from build123d import *

# Parameters (mm, degrees)
SKETCH_1_R               = 6.65
EXTRUDE_1_DEPTH          = 20
SKETCH_2_R               = 1.5
CUT_EXTRUDE_1_DEPTH      = 35.073450075
SKETCH_3_R               = 1.45
CUT_EXTRUDE_2_DEPTH      = 10
PATTERN_CIRCULAR_1_COUNT = 2
PATTERN_CIRCULAR_1_ANGLE = 90
F_1_THE_OTHER_WAY_COUNT  = 2
F_1_THE_OTHER_WAY_ANGLE  = 90
SKETCH_4_R               = 4.65
EXTRUDE_2_DEPTH          = 2
FILLET_1_R               = 2


with BuildPart() as part:
    # 草图1 → 凸台-拉伸1 (new body)
    with BuildSketch(Plane(origin=(0, 0, 0), x_dir=(1, 0, 0), z_dir=(0, 1, 0))):
        with BuildLine():
            Line((-11, 0), (-11, -8))
            Line((-11, -8), (-20, -8))
            Line((-20, -8), (-20, -13))
            Line((-20, -13), (20, -13))
            Line((20, -13), (20, -8))
            Line((20, -8), (11, -8))
            Line((11, -8), (11, 0))
            ThreePointArc((11, 0), (0, 11), (-11, 0))
        make_face()
        with Locations(Location((0, 0, 0), (0, 0, 270))):
            Circle(SKETCH_1_R, mode=Mode.SUBTRACT)
    extrude(amount=EXTRUDE_1_DEPTH)

    # 草图2 → 切除-拉伸1 (cut, through all)
    with BuildSketch(Plane(origin=(0, 0, 8), x_dir=(-1, 0, 0), z_dir=(0, 0, -1))):
        with Locations((15.5, 5)):
            Circle(SKETCH_2_R)
        with Locations(Location((15.5, 15, 0), (0, 0, 180))):
            Circle(SKETCH_2_R)
        with Locations((-15.5, 15)):
            Circle(SKETCH_2_R)
        with Locations(Location((-15.5, 5, 0), (0, 0, 180))):
            Circle(SKETCH_2_R)
    extrude(amount=-CUT_EXTRUDE_1_DEPTH, mode=Mode.SUBTRACT)

    # 草图3 → 切除-拉伸2 (cut)
    with BuildSketch(Plane(origin=(0, 0, -11), x_dir=(-1, 0, 0), z_dir=(0, 0, -1))):
        with Locations((0, 6)):
            Circle(SKETCH_3_R)
        with Locations((0, 14)):
            Circle(SKETCH_3_R)
    cut_extrude_2 = extrude(amount=-CUT_EXTRUDE_2_DEPTH, mode=Mode.SUBTRACT)

    # 阵列(圆周)1: 切除-拉伸2 ×2 about axis
    pattern_circular_1_axis = Axis((0, 20, 0), (0, -1, 0))
    for i in range(1, PATTERN_CIRCULAR_1_COUNT):
        add(cut_extrude_2.rotate(pattern_circular_1_axis, i * PATTERN_CIRCULAR_1_ANGLE / (PATTERN_CIRCULAR_1_COUNT - 1)), mode=Mode.SUBTRACT)

    # 1 the other way: 切除-拉伸2 ×2 about axis
    f_1_the_other_way_axis = Axis((0, 20, 0), (0, 1, 0))
    for i in range(1, F_1_THE_OTHER_WAY_COUNT):
        add(cut_extrude_2.rotate(f_1_the_other_way_axis, i * F_1_THE_OTHER_WAY_ANGLE / (F_1_THE_OTHER_WAY_COUNT - 1)), mode=Mode.SUBTRACT)

    # 草图4 → 凸台-拉伸2 (add)
    with BuildSketch(Plane(origin=(0, 20, 0), x_dir=(1, 0, 0), z_dir=(0, 1, 0))):
        with BuildLine():
            Line((20, -8), (11, -8))
            Line((11, -8), (11, 0))
            ThreePointArc((11, 0), (0, 11), (-11, 0))
            Line((-11, 0), (-11, -8))
            Line((-11, -8), (-20, -8))
            Line((-20, -8), (-20, -13))
            Line((-20, -13), (20, -13))
            Line((20, -13), (20, -8))
        make_face()
        with Locations(Location((0, 0, 0), (0, 0, 270))):
            Circle(SKETCH_4_R, mode=Mode.SUBTRACT)
    extrude(amount=EXTRUDE_2_DEPTH)

    # 圆角1
    fillet_1_edges = [part.edges().sort_by_distance(p)[0] for p in [
        (20, 0, 10.5),
        (-20, 0, 10.5),
        (20, 22, 10.5),
        (-20, 22, 10.5),
    ]]
    fillet(fillet_1_edges, radius=FILLET_1_R)


solid = part.part
The model under review builds one solid part; all positions refer to its coordinate system, in mm. A direction names the side the tool comes from. Give positions to 0.01 mm unless a question says otherwise; leave off trailing zeros. Order: outer loops, then holes, each group sorted by start corner. A loop starts at its lowest first (then second) coordinate and runs counter-clockwise, first axis right, second up. Notation, with made-up numbers: M 45,41.5 L 88,41.5 A16 ccw 88,68.5 Z; hole C 19.5,-29 d3. An arc over 180 degrees is marked long. One line per question, with ' | ' between items. Start each with the question number.
1) For faces 5 (the face through (-15, 11, 8)), 6 (the face through (11, 11, 4)), 7 (the face through (1.397, 20.986, 4.435)), 8 (the face through (0.189, 15.438, -8.777)), 9 (the face through (-5, 20, 1)), list the 3-axis set-ups (+Z, -Z, +X, -X, +Y, -Y) from which the entire face can be reached by the end or side of a thin tool; tool diameter is ignored.
2) Consider section D-D, the plane x = 15.5. Give the boundary of the cut face in (y, z), then the cut area to 3 significant figures.
3) Consider section A-A, the plane x = 0. Give the boundary of the cut face in (y, z), then the cut area to 3 significant figures.
4) Consider section C-C, the plane y = 12. Give the boundary of the cut face in (x, z).
5) Consider section B-B, the plane z = 9. Give the boundary of the cut face in (x, y).
6) Clearance check with flat-ended pins moving along their axes: P1, Ø4, axis at x = -1.5, z = -1, coming from the -Y side; P2, Ø3.5, axis at x = -15.5, y = 5, coming from the -Z side; P3, Ø4, axis at x = 10.5, y = 18, coming from the -Z side; P4, Ø2, axis at y = 8, z = 1.5, coming from the +X side. State where each tip first meets the part, or that it passes through.
7) Mouldability with a two-part tool opening along X and no side actions: class faces 1 (the face through (-8.774, 7.438, -0.189)), 2 (the face through (-14, 5, 10)), 3 (the face through (19.4, 0.57, 10.46)), 4 (the face through (-5.9, 9.86, 3.07)) as pulls with the +X half, pulls with the -X half, needs draft (parallel to the pull), parting line crosses it, or undercut.
8) Wall thickness on L1, parallel to Y at x = -15.5, z = 9.4; L2, parallel to Y at x = 0, z = -8.25; L3, parallel to X at y = 3.75, z = 0.25: over which ranges is each line inside the solid? List them lowest first. Write a range as from..to.
Found:
1) face 5: -Z, -X, +Y, -Y | face 6: -Z, +X, +Y, -Y | face 7: +Y, -Y | face 8: -Z | face 9: -Y
2) outline: M 0,8 L 3.5,8 L 3.5,13 L 0,13 Z; M 6.5,8 L 13.5,8 L 13.5,13 L 6.5,13 Z; M 16.5,8 L 22,8 L 22,13 L 16.5,13 Z | area: 80.0 mm²
3) outline: M 0,-11 L 4.55,-11 L 4.55,-6.65 L 0,-6.65 Z; M 0,6.65 L 20,6.65 L 20,4.65 L 22,4.65 L 22,13 L 0,13 Z; M 7.45,-11 L 12.55,-11 L 12.55,-6.65 L 7.45,-6.65 Z; M 15.45,-11 L 22,-11 L 22,-4.65 L 20,-4.65 L 20,-6.65 L 15.45,-6.65 Z | area: 218 mm²
4) outline: M -20,8 L -11,8 L -11,0 A11 ccw 11,0 L 11,8 L 20,8 L 20,13 L -20,13 Z; hole C 0,0 d13.3
5) outline: M -20,2 A2 ccw -18,0 L 18,0 A2 ccw 20,2 L 20,20 A2 ccw 18,22 L -18,22 A2 ccw -20,20 Z; hole C -15.5,5 d3; hole C -15.5,15 d3; hole C 15.5,5 d3; hole C 15.5,15 d3
6) P1: passes through | P2: stops at z = 8 | P3: stops at z = -6.98 | P4: stops at x = 11
7) face 1: needs draft | face 2: undercut | face 3: pulls with the +X half | face 4: undercut
8) L1: y = 0..3.5, 6.5..13.5, 16.5..22 | L2: y = 0..4.55, 7.45..12.55, 15.45..22 | L3: x = -11..-6.65, 6.65..11
